from build123d import *

# Parameters (mm, degrees)
BOSS_EXTRUDE1_DEPTH = 3
CUT_EXTRUDE1_REACH  = 265.453
SKETCH2_R           = 1.5
LPATTERN2_COUNT     = 3
LPATTERN2_PITCH     = 63.5
CUT_EXTRUDE2_REACH  = 265.453
SKETCH3_R           = 1.5
CUT_EXTRUDE3_REACH  = 265.453
SKETCH4_R           = 1.5
CUT_EXTRUDE4_REACH  = 265.453
SKETCH5_R           = 1.5


with BuildPart() as part:
    # Sketch1 → Boss-Extrude1 (new body)
    with BuildSketch(Plane.XY):
        Polygon((0, 0), (-195.53, 0), (-195.53, 77.54), (-122.53, 77.54), (-23.54, 176.54), (0, 176.54), align=None)
    extrude(amount=BOSS_EXTRUDE1_DEPTH)

    # Sketch2 → Cut-Extrude1 (cut, up to next)
    with BuildSketch(Plane.XY.offset(3), mode=Mode.PRIVATE) as cut_extrude1_sk1:
        with Locations((-24.04, 166.4)):
            Circle(SKETCH2_R)
    cut_extrude1_tool1 = extrude(cut_extrude1_sk1.sketch, amount=-CUT_EXTRUDE1_REACH, mode=Mode.PRIVATE) & part.part
    cut_extrude1 = cut_extrude1_tool1.solids().sort_by_distance((-24.04, 166.4, 3))[0]
    add(cut_extrude1, mode=Mode.SUBTRACT)

    # LPattern2: Cut-Extrude1 ×3
    with Locations(*[Vector(-0.707071066017225, -0.707142494552028, 0) * (i * LPATTERN2_PITCH) for i in range(1, LPATTERN2_COUNT)]):
        add(cut_extrude1, mode=Mode.SUBTRACT)

    # Sketch3 → Cut-Extrude2 (cut, up to next)
    with BuildSketch(Plane.XY.offset(3), mode=Mode.PRIVATE) as cut_extrude2_sk1:
        with Locations((-18, 10)):
            Circle(SKETCH3_R)
    cut_extrude2_tool1 = extrude(cut_extrude2_sk1.sketch, amount=-CUT_EXTRUDE2_REACH, mode=Mode.PRIVATE) & part.part
    # Sketch3 → Cut-Extrude2 (cut, up to next)
    with BuildSketch(Plane.XY.offset(3), mode=Mode.PRIVATE) as cut_extrude2_sk2:
        with Locations((-85.5, 10)):
            Circle(SKETCH3_R)
    cut_extrude2_tool2 = extrude(cut_extrude2_sk2.sketch, amount=-CUT_EXTRUDE2_REACH, mode=Mode.PRIVATE) & part.part
    # Sketch3 → Cut-Extrude2 (cut, up to next)
    with BuildSketch(Plane.XY.offset(3), mode=Mode.PRIVATE) as cut_extrude2_sk3:
        with Locations((-153, 10)):
            Circle(SKETCH3_R)
    cut_extrude2_tool3 = extrude(cut_extrude2_sk3.sketch, amount=-CUT_EXTRUDE2_REACH, mode=Mode.PRIVATE) & part.part
    add(cut_extrude2_tool1.solids().sort_by_distance((-18, 10, 3))[0], mode=Mode.SUBTRACT)
    add(cut_extrude2_tool2.solids().sort_by_distance((-85.5, 10, 3))[0], mode=Mode.SUBTRACT)
    add(cut_extrude2_tool3.solids().sort_by_distance((-153, 10, 3))[0], mode=Mode.SUBTRACT)

    # Sketch4 → Cut-Extrude3 (cut, up to next)
    with BuildSketch(Plane.XY.offset(3), mode=Mode.PRIVATE) as cut_extrude3_sk1:
        with Locations((-150.995, 67.54)):
            Circle(SKETCH4_R)
    cut_extrude3_tool1 = extrude(cut_extrude3_sk1.sketch, amount=-CUT_EXTRUDE3_REACH, mode=Mode.PRIVATE) & part.part
    add(cut_extrude3_tool1.solids().sort_by_distance((-150.995, 67.54, 3))[0], mode=Mode.SUBTRACT)

    # Sketch5 → Cut-Extrude4 (cut, up to next)
    with BuildSketch(Plane.XY.offset(3), mode=Mode.PRIVATE) as cut_extrude4_sk1:
        with Locations((-8, 85.01)):
            Circle(SKETCH5_R)
    cut_extrude4_tool1 = extrude(cut_extrude4_sk1.sketch, amount=-CUT_EXTRUDE4_REACH, mode=Mode.PRIVATE) & part.part
    add(cut_extrude4_tool1.solids().sort_by_distance((-8, 85.01, 3))[0], mode=Mode.SUBTRACT)


solid = part.part
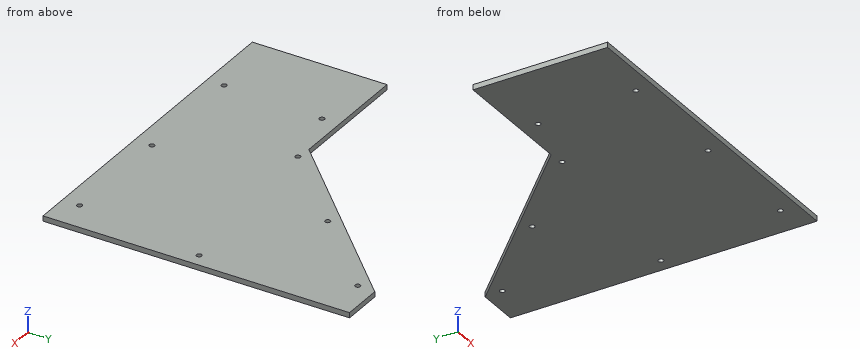
Input: part model. Units: mm. Frame: model coordinates. Round coordinates to 2 decimals unless told otherwise and drop trailing zeros. Order: outer loops, then holes, each group sorted by start corner. A loop starts at its lowest first (then second) coordinate and runs counter-clockwise, first axis right, second up. Notation, with made-up numbers: (-5.75, -19) - (-0.75, -19) arc R16 ccw to (-0.75, -9) - close; hole circle Ø9 at (19.25, 21). An arc over 180 degrees is marked (long way). Answer as a JSON object with one key per item and string values. Group by question number.
(1) Cut plane B-B (x = -175.5). Return loops of the section in (y, z), then the cut area to 3 significant figures.
(2) Cut plane C-C (y = 106.5). Return loops of the section in (x, z).
(3) Material intervals for probe 1 along Y at (x, z) = (-18, 2.3); probe 2 along X at (y, z) = (67.54, 0.8) (3 decimals); probe 3 along Y at (x, z) = (-85.5, 1.8), sorted ascending. Write a range as from..to.
(4) Pin query (flat end, axial travel): P1, Ø1.8, axis at x = -8, y = 85.01, coming from the -Z side; P2, Ø3.5, axis at x = -150.995, y = 67.54, coming from the +Z side; P3, Ø1.5, axis at x = -155, z = 1, coming from the +Y side; P4, Ø1, axis at x = -79, z = 1, coming from the +Y side. Return the tip coordinate at first contact, or that it passes through.
(5) Cut plane A-A (z = 1.35). Count the separate pieces of the cut face and the enclosed holes in it, then the cut area to 3 significant figures.
Here are the results:
{
 "1": {"outline": "(0, 0) - (77.54, 0) - (77.54, 3) - (0, 3) - close", "area": "233 mm^2"},
 "2": {"outline": "(-93.57, 0) - (0, 0) - (0, 3) - (-93.57, 3) - close"},
 "3": {"probe 1": "y = 0..8.5, 11.5..176.54", "probe 2": "x = -195.53..-152.495, -149.495..0", "probe 3": "y = 0..8.5, 11.5..114.57"},
 "4": {"P1": "passes through", "P2": "stops at z = 3", "P3": "stops at y = 77.54", "P4": "stops at y = 121.57"},
 "5": {"separate pieces": "1", "enclosed holes": "8", "area": "22,300 mm^2"}
}
